from build123d import *

# Parameters (mm, degrees)
F0_W     = 300
F0_H     = 300
F1_DEPTH = 150
F2_T     = -12
F3_W     = 276
F3_H     = 12
F4_DEPTH = 288
F5_W     = 276
F5_H     = 12
F6_DEPTH = 288


with BuildPart() as f1:
    # F0 (on Front) → F1 (new body, symmetric)
    with BuildSketch(Plane.XZ):
        Rectangle(F0_W, F0_H)
    extrude(amount=F1_DEPTH, both=True)

    # F2
    f2_openings = [f1.faces().sort_by_distance(p)[0] for p in [
        (0, -150, 0),
    ]]
    offset(amount=F2_T, openings=f2_openings)

    # F3 (on face) → F4 (join)
    with BuildSketch(Plane.XZ.offset(150)):
        with Locations((0, 23.6249938158)):
            Rectangle(F3_W, F3_H)
    extrude(amount=-F4_DEPTH)

    # F5 (on face) → F6 (join)
    with BuildSketch(Plane.XZ.offset(150)):
        with Locations((0, -54.6922665407)):
            Rectangle(F5_W, F5_H)
    extrude(amount=-F6_DEPTH)


solid = f1.part
Could you check a few things on this model? Use its own coordinates, in mm. A direction names the side the tool comes from. Round coordinates to 2 decimals unless told otherwise and drop trailing zeros. Order: outer loops, then holes, each group sorted by start corner. A loop starts at its lowest first (then second) coordinate and runs counter-clockwise, first axis right, second up.
Q1. Imagine slicing it at B-B, the plane y = 120. List the corners of the cut face in (x, z) for me (3 decimals), then the cut area to 3 significant figures.
Geometry says:
outline: (-150, -150) - (150, -150) - (150, 150) - (-150, 150) - close; hole (-138, -138) - (138, -138) - (138, -60.692) - (-138, -60.692) - close; hole (-138, -48.692) - (138, -48.692) - (138, 17.625) - (-138, 17.625) - close; hole (-138, 29.625) - (138, 29.625) - (138, 138) - (-138, 138) - close
area: 20,400 mm2
Q2. Imagine slicing it at A-A, the plane z = 69. List the corners of the cut face in (x, y) for me.
Geometry says:
outline: (-150, -150) - (-138, -150) - (-138, 138) - (138, 138) - (138, -150) - (150, -150) - (150, 150) - (-150, 150) - close
Q3. I'm going to push a flat-ended pin straight in: P1, Ø5, axis at x = -6, z = -19, coming from the -Y side. Where does the tip first touch, or does it pass through?
Geometry says:
P1: stops at y = 138
Q4. Imagine slicing it at C-C, the plane x = -131. List the corners of the cut face in (y, z) for me (3 decimals).
Geometry says:
outline: (-150, -150) - (150, -150) - (150, 150) - (-150, 150) - (-150, 138) - (138, 138) - (138, 29.625) - (-150, 29.625) - (-150, 17.625) - (138, 17.625) - (138, -48.692) - (-150, -48.692) - (-150, -60.692) - (138, -60.692) - (138, -138) - (-150, -138) - close
Q5. Which directions (+Z, -Z, +X, -X, +Y, -Y) give clear straight access to the entire face, cutting with the end or side of a thin tool? Please do faces 4 (the face through (-2, -8, 17.625)), 5 (the face through (-150, -2, -2)).
Geometry says:
face 4: -Y
face 5: +Z, -Z, -X, +Y, -Y
Q6. Thinking about a two-plate mould opening in Z: for faces 1 (the face through (-2, 138, -99)), 2 (the face through (-2, -2, -150)), 3 (the face through (-2, -2, 150)), which applies, released by +Z, released by -Z, zero draft, split by the parting line, or undercut?
Geometry says:
face 1: undercut
face 2: released by -Z
face 3: released by +Z
Q7. Please list where these lines run through material, in increasing order: probe 1 along Z at (x, y) = (13, 78) (3 decimals); probe 2 along X at (y, z) = (63.5, -25.5); probe 3 along Y at (x, z) = (-79.5, -43).
Geometry says:
probe 1: z = -150 to -138, -60.692 to -48.692, 17.625 to 29.625, 138 to 150
probe 2: x = -150 to -138, 138 to 150
probe 3: y = 138 to 150
